CAD build for the part. Positions are in the model's coordinates, mm. A direction names the side the tool comes from. Round coordinates to 2 decimals unless told otherwise and drop trailing zeros. Loops run counter-clockwise (first coordinate to the right, second up) from the corner with the lowest first, then second, coordinate; pieces in that order, holes last. Notation, with made-up numbers: M 74,66 L 113,66 A16 ccw 113,76 Z; hole C -14,-36 d8. An arc over 180 degrees is marked long. Use a Markdown table: item, result. Add a question column.
(1) Flat gauge pins, fed straight in: P1, Ø8, axis at x = -12.5, z = 3.5, coming from the +Y side; P2, Ø4, axis at x = 9.5, y = -1, coming from the +Z side; P3, Ø0.9, axis at x = -36, y = -3.5, coming from the +Z side; P4, Ø5, axis at x = -4, y = -2, coming from the +Z side. Where does each tip first touch, or does it go through?
(2) Band-saw the part on B-B, the plane z = -1.5. Write the cut outline in (x, y).
(3) Which spindle directions (+Z, -Z, +X, -X, +Y, -Y) get a long thin tool onto all of the face, cutting with end or side? Do faces 5 (the face through (-20, -8.5, -1)), 6 (the face through (-27.9, 0, -2.7)), 7 (the face through (-1, -6, 0)), 8 (the face through (-37.51, -4.26, 15.81)), 9 (the face through (-22, 1.7, -1)). Say none if no direction does.
(4) Band-saw the part on C-C, the plane x = 19. Write the cut outline in (y, z), and give its area (4 significant figures).
(5) Two-plate mould, pull along X, no slides. Class faces 1 (the face through (27.9, 0, -2.7)), 2 (the face through (-16.3, 0, -1.3)), 3 (the face through (-20, 8.5, -1)), 4 (the face through (-44, 0, 8)): released by +X, released by -X, zero draft, split by the parting line, or undercut.
(6) Band-saw the part on A-A, the plane y = 0. Write the cut outline in (x, z).
(7) Wall check: L1, parallel to Y at x = 4, z = -1.5; L2, parallel to X at y = -0.75, z = 4; L3, parallel to Z at x = -19.5, y = 7.5. Give the ranges that are in metal, low to high.
(8) Band-saw the part on D-D, the plane z = 14.5. Write the cut outline in (x, y).
from build123d import *

# Parameters (mm, degrees)
PAD_DEPTH       = 8.5
POCKET_DEPTH    = 24.001
POCKET001_DEPTH = 8.5
CHAMFER_SIZE    = 1.5
CHAMFER001_SIZE = 1.5


with BuildPart() as part:
    # Sketch → Pad (new body, symmetric)
    with BuildSketch(Plane.XZ):
        Polygon((-44, -4), (-44, 20), (-34, 20), (-34, 0), (33, 0), (33, -4), align=None)
    extrude(amount=PAD_DEPTH, both=True)

    # Sketch001 → Pocket (cut, through all)
    with BuildSketch(Plane(origin=(0, 0, -4), x_dir=(1, 0, 0), z_dir=(0, 0, -1))):
        with BuildLine():
            ThreePointArc((-26, 1.7), (-27.7, 0), (-26, -1.7))
            Line((-26, -1.7), (-18, -1.7))
            ThreePointArc((-18, -1.7), (-16.3, 0), (-18, 1.7))
            Line((-26, 1.7), (-18, 1.7))
        make_face()
        with BuildLine():
            ThreePointArc((-4, 5.5), (-9.5, 0), (-4, -5.5))
            Line((-4, -5.5), (4, -5.5))
            ThreePointArc((4, -5.5), (9.5, 0), (4, 5.5))
            Line((-4, 5.5), (4, 5.5))
        make_face()
        with BuildLine():
            ThreePointArc((18, 1.7), (16.3, 0), (18, -1.7))
            Line((18, -1.7), (26, -1.7))
            ThreePointArc((26, -1.7), (27.7, 0), (26, 1.7))
            Line((18, 1.7), (26, 1.7))
        make_face()
    extrude(amount=-POCKET_DEPTH, mode=Mode.SUBTRACT)

    # Sketch006 → Pocket001 (cut)
    with BuildSketch(Plane(origin=(0, 0, 20), x_dir=(-1, 0, 0), z_dir=(0, 0, 1))):
        Polygon((34.748284, 6.431895), (37.232557, 6.711868), (37.792504, 1.743321), (35.30823, 1.463348), align=None)
        Polygon((35.30823, -1.463348), (37.792504, -1.743321), (37.232557, -6.711868), (34.748284, -6.431895), align=None)
    extrude(amount=-POCKET001_DEPTH, mode=Mode.SUBTRACT)

    # Chamfer
    chamfer_edges = [part.edges().sort_by_distance(p)[0] for p in [
        (22, 1.7, -4),
    ]]
    chamfer(chamfer_edges, length=CHAMFER_SIZE)

    # Chamfer001
    chamfer001_edges = [part.edges().sort_by_distance(p)[0] for p in [
        (-22, 1.7, -4),
    ]]
    chamfer(chamfer001_edges, length=CHAMFER001_SIZE)


solid = part.part
Return value:
| question | item | result |
|---|---|---|
| 1 | P1 | y = 8.5 |
| 1 | P2 | z = 0 |
| 1 | P3 | z = 11.5 |
| 1 | P4 | through |
| 2 | outline | M -44,-8.5 L 33,-8.5 L 33,8.5 L -44,8.5 Z; hole M -26,-1.7 L -18,-1.7 A1.7 ccw -18,1.7 L -26,1.7 A1.7 ccw Z; hole M -4,-5.5 L 4,-5.5 A5.5 ccw 4,5.5 L -4,5.5 A5.5 ccw Z; hole M 18,-1.7 L 26,-1.7 A1.7 ccw 26,1.7 L 18,1.7 A1.7 ccw Z |
| 3 | face 5 | +Z, -Z, +X, -X, -Y |
| 3 | face 6 | -Z |
| 3 | face 7 | +Z, +X, +Y, -Y |
| 3 | face 8 | +Z |
| 3 | face 9 | +Z, -Z |
| 4 | outline | M -8.5,-4 L -3.2,-4 L -1.7,-2.5 L -1.7,0 L -8.5,0 Z; M 1.7,-2.5 L 3.2,-4 L 8.5,-4 L 8.5,0 L 1.7,0 Z |
| 4 | area | 52.15 mm^2 |
| 5 | face 1 | undercut |
| 5 | face 2 | undercut |
| 5 | face 3 | zero draft |
| 5 | face 4 | released by -X |
| 6 | outline | M -44,-4 L -29.2,-4 L -27.7,-2.5 L -27.7,0 L -34,0 L -34,20 L -44,20 Z; M -16.3,-2.5 L -14.8,-4 L -9.5,-4 L -9.5,0 L -16.3,0 Z; M 9.5,-4 L 14.8,-4 L 16.3,-2.5 L 16.3,0 L 9.5,0 Z; M 27.7,-2.5 L 29.2,-4 L 33,-4 L 33,0 L 27.7,0 Z |
| 7 | L1 | -8.5 to -5.5, 5.5 to 8.5 |
| 7 | L2 | -44 to -34 |
| 7 | L3 | -4 to 0 |
| 8 | outline | M -44,-8.5 L -34,-8.5 L -34,8.5 L -44,8.5 Z; hole M -37.79,-1.74 L -37.23,-6.71 L -34.75,-6.43 L -35.31,-1.46 Z; hole M -37.79,1.74 L -35.31,1.46 L -34.75,6.43 L -37.23,6.71 Z |
